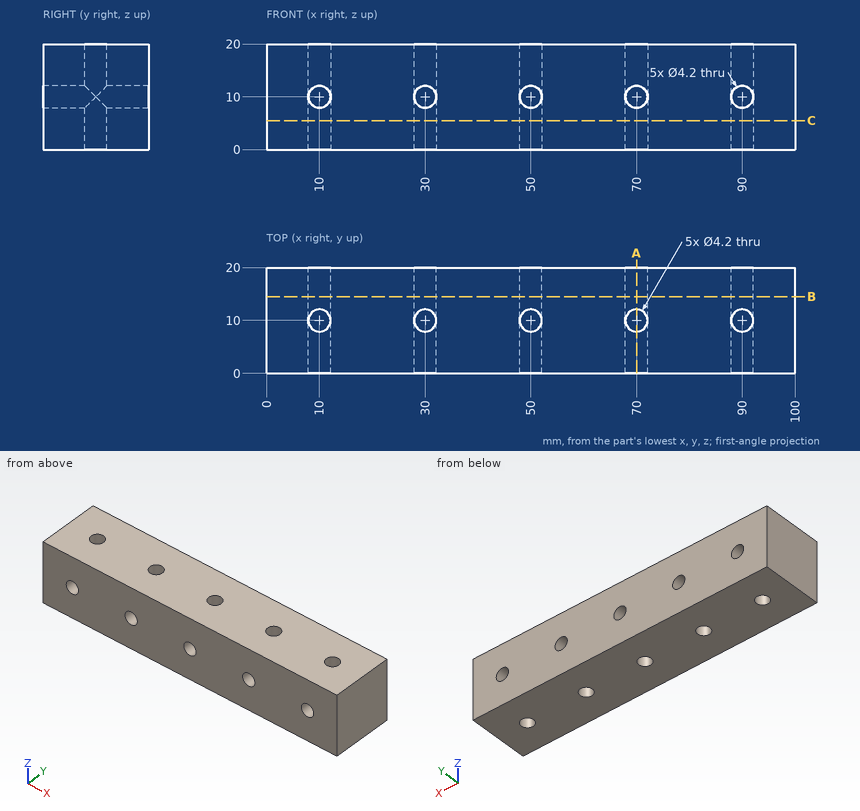
Check sheet for the drawn part. Datum: minimum x, y, z corner. Units: mm. Coordinates: 2 decimals unless noted, no trailing zeros. Loops run counter-clockwise (first coordinate to the right, second up) from the corner with the lowest first, then second, coordinate; pieces in that order, holes last. Notation, with made-up numbers: (17.5, 14) -> (36.5, 14) arc R13 cw to (36.5, 31) -> close; hole circle Ø3 at (-14, 10). An arc over 180 degrees is marked (long way). Write each question's results on one line, items separated by ' | '.
Item 1: Section check B-B, the plane y = 14.5. Enter the section's corners in (x, z).
Found:
outline: (0, 0) -> (100, 0) -> (100, 20) -> (0, 20) -> close; hole circle Ø4.2 at (10, 10); hole circle Ø4.2 at (30, 10); hole circle Ø4.2 at (50, 10); hole circle Ø4.2 at (70, 10); hole circle Ø4.2 at (90, 10)
Item 2: Section check A-A, the plane x = 70. Enter the section's corners in (y, z).
Found:
outline: (0, 0) -> (7.9, 0) -> (7.9, 7.9) -> (0, 7.9) -> close; (0, 12.1) -> (7.9, 12.1) -> (7.9, 20) -> (0, 20) -> close; (12.1, 0) -> (20, 0) -> (20, 7.9) -> (12.1, 7.9) -> close; (12.1, 12.1) -> (20, 12.1) -> (20, 20) -> (12.1, 20) -> close
Item 3: Material ranges on L1, parallel to X at y = 10, z = 14.5; L2, parallel to Z at x = 10, y = 5, recorded low to high.
Found:
L1: x = 0 to 7.9, 12.1 to 27.9, 32.1 to 47.9, 52.1 to 67.9, 72.1 to 87.9, 92.1 to 100 | L2: z = 0 to 7.9, 12.1 to 20
Item 4: Gauge pin test, flat ends, axial feed: pin 1 (2.5 mm diameter, centred on x = 70, z = 10, fed in from +Y); pin 2 (5 mm diameter, centred on x = 90, y = 10, fed in from +Z). Record the tip position at first contact, or that the pin passes through.
Found:
pin 1: passes through | pin 2: stops at z = 20
